Design review of the part shown in the three views and the two pictorial views. Dimensions are in mm from the part's minimum x, y and z. Round coordinates to 2 decimals unless told otherwise and drop trailing zeros. Order: outer loops, then holes, each group sorted by start corner. A loop starts at its lowest first (then second) coordinate and runs counter-clockwise, first axis right, second up.
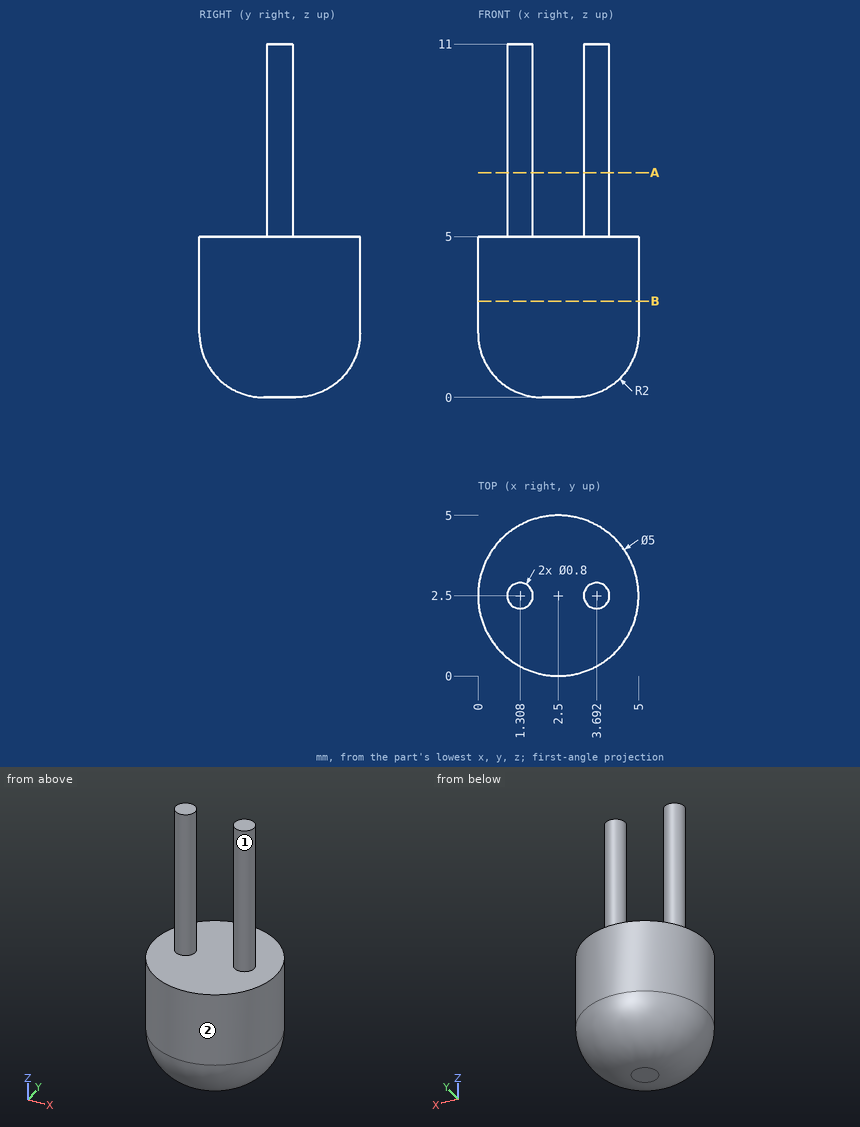
1) To check wall thickness, follow line 1 along Z through (x, y) = (2.25, 2.5); line 2 along X through (y, z) = (2.2, 9) (1 decimal). State the ranges of each line that lie inside material, in increasing order.
Results:
line 1: z = 0 to 5
line 2: x = 1 to 1.6, 3.4 to 4
2) Take a section at B-B on z = 3. Give the boundary of the cut face in (x, y), plus the area to 3 significant figures.
Results:
outline: circle Ø5 at (2.5, 2.5)
area: 19.6 mm2
3) Clearance check with flat-ended pins moving along their axes: P1, Ø2, axis at x = 4.5, y = 1, coming from the +Z side; P2, Ø1, axis at x = 3.5, z = 9.5, coming from the -Y side; P3, Ø3, axis at x = 1, y = 1, coming from the -Z side. State where each tip first meets the part, or that it passes through.
Results:
P1: stops at z = 5
P2: stops at y = 2.1
P3: stops at z = 0
4) Take a section at A-A on z = 7. Give the boundary of the cut face in (x, y).
Results:
outline: circle Ø0.8 at (1.31, 2.5); circle Ø0.8 at (3.69, 2.5)
5) The part is to be moulded in two halves that separate along X. For the marked faces 1 and 2, say which applies: released by +X, released by -X, zero draft, split by the parting line, or undercut.
Results:
face 1: undercut
face 2: split by the parting line
